Check sheet for the modelled part. Datum: model origin and axes. Units: mm. A direction names the side the tool comes from. Round coordinates to 2 decimals unless told otherwise and drop trailing zeros. Write each loop counter-clockwise with the first axis right and the second up, starting at its lowest first coordinate (ties: lowest second). Pieces come first, ordered by that corner, then holes. Notation, with made-up numbers: M 49.25,-17.5 L 74.25,-17.5 A27 ccw 74.25,2.5 Z; hole C 0.5,9.5 d4. An arc over 180 degrees is marked long. One line per item, written item: value.
from build123d import *

# Parameters (mm, degrees)
SKETCH_R        = 2.5
SKETCH_R_2      = 1.6
PAD_DEPTH       = 65
PAD001_DEPTH    = 1.5
PAD002_DEPTH    = 5
SKETCH003_W     = 2
SKETCH003_H     = 7
POCKET_DEPTH    = 7.001
SKETCH004_R     = 1.1
POCKET001_DEPTH = 7.001
SKETCH006_W     = 2.5
SKETCH006_H     = 11
POCKET002_DEPTH = 8.001
SKETCH005_W     = 2.5
SKETCH005_H     = 11
POCKET003_DEPTH = 8.001
POCKET004_DEPTH = 7.001


with BuildPart() as part:
    # Sketch → Pad (new body)
    with BuildSketch(Plane.XY):
        Circle(SKETCH_R)
        Circle(SKETCH_R_2, mode=Mode.SUBTRACT)
    extrude(amount=PAD_DEPTH)

    # Sketch001 (on Face3 of Pad) → Pad001 (join)
    with BuildSketch(Plane(origin=(0, 0, 7), x_dir=(1, 0, 0), z_dir=(0, 0, -1))):
        with BuildLine():
            Line((-2, 4), (2, 4))
            ThreePointArc((4, 2), (3.414214, 3.414214), (2, 4))
            Line((4, 2), (4, -2))
            ThreePointArc((2, -4), (3.414214, -3.414214), (4, -2))
            Line((2, -4), (-2, -4))
            ThreePointArc((-4, -2), (-3.414214, -3.414214), (-2, -4))
            Line((-4, -2), (-4, 2))
            ThreePointArc((-2, 4), (-3.414214, 3.414214), (-4, 2))
        make_face()
    extrude(amount=-PAD001_DEPTH)

    # Sketch002 (on Face16 of Pad001) → Pad002 (join)
    with BuildSketch(Plane.XY.offset(65)):
        with BuildLine():
            Line((-1, 3), (1, 3))
            ThreePointArc((3, 1), (2.414214, 2.414214), (1, 3))
            Line((3, 1), (3, -1))
            ThreePointArc((1, -3), (2.414214, -2.414214), (3, -1))
            Line((1, -3), (-1, -3))
            ThreePointArc((-3, -1), (-2.414214, -2.414214), (-1, -3))
            Line((-3, -1), (-3, 1))
            ThreePointArc((-1, 3), (-2.414214, 2.414214), (-3, 1))
        make_face()
    extrude(amount=PAD002_DEPTH)

    # Sketch003 (on Face10 of Pad002) → Pocket (cut, through all)
    with BuildSketch(Plane.YZ.offset(3)):
        with Locations((0, 66.5)):
            Rectangle(SKETCH003_W, SKETCH003_H)
    extrude(amount=-POCKET_DEPTH, mode=Mode.SUBTRACT)

    # Sketch004 (on Face3 of Pocket) → Pocket001 (cut, through all)
    with BuildSketch(Plane.XZ.offset(3)):
        with Locations((0, 67.5)):
            Circle(SKETCH004_R)
    extrude(amount=-POCKET001_DEPTH, mode=Mode.SUBTRACT)

    # Sketch006 (on Face28 of Pocket001) → Pocket002 (cut, through all)
    with BuildSketch(Plane.XZ.offset(4)):
        with Locations((0, 16)):
            Rectangle(SKETCH006_W, SKETCH006_H)
        with Locations((0, 29)):
            Rectangle(SKETCH006_W, SKETCH006_H)
        with Locations((0, 42)):
            Rectangle(SKETCH006_W, SKETCH006_H)
        with Locations((0, 55)):
            Rectangle(SKETCH006_W, SKETCH006_H)
    extrude(amount=-POCKET002_DEPTH, mode=Mode.SUBTRACT)

    # Sketch005 (on Face31 of Pocket001) → Pocket003 (cut, through all)
    with BuildSketch(Plane.YZ.offset(4)):
        with Locations((0, 16)):
            Rectangle(SKETCH005_W, SKETCH005_H)
        with Locations((0, 29)):
            Rectangle(SKETCH005_W, SKETCH005_H)
        with Locations((0, 42)):
            Rectangle(SKETCH005_W, SKETCH005_H)
        with Locations((0, 55)):
            Rectangle(SKETCH005_W, SKETCH005_H)
    extrude(amount=-POCKET003_DEPTH, mode=Mode.SUBTRACT)

    # Sketch007 (on Face5 of Pocket003) → Pocket004 (cut, through all)
    with BuildSketch(Plane.XZ.offset(3)):
        with BuildLine():
            ThreePointArc((3, 67.251006), (2.034513, 69.208821), (0, 70))
            Line((0, 70), (3, 70))
            Line((3, 67.251006), (3, 70))
        make_face()
    extrude(amount=-POCKET004_DEPTH, mode=Mode.SUBTRACT)


solid = part.part
Q1. Scan lines: line 1 (Z direction, x = 1, y = 2.5); line 2 (X direction, y = 0, z = 4.75). Record each from-to range of solid material in increasing order. Write a range as [from, to].
Completed:
line 1: [7, 8.5], [65, 67.04], [67.96, 69.83]
line 2: [-2.5, -1.6], [1.6, 2.5]
Q2. Depth check by flat-ended pin: P1, Ø2, axis at x = 0, z = 66.5, coming from the -Y side; P2, Ø0.7, axis at y = -1.5, z = 52.5, coming from the +X side; P3, Ø3, axis at x = -2.5, z = 36.5, coming from the -Y side. Enter the tip coordinate at first touch or a pass-through.
Completed:
P1: y = -3
P2: x = 2.17
P3: y = -2.29
Q3. Sectioned sample at A-A on z = 20.5. Enter the section's corners in (x, y).
Completed:
outline: M -2.17,-1.25 A2.5 ccw -1.25,-2.17 L -1.25,-1.25 Z; M -2.17,1.25 L -1.25,1.25 L -1.25,2.17 A2.5 ccw Z; M 1.25,-2.17 A2.5 ccw 2.17,-1.25 L 1.25,-1.25 Z; M 1.25,1.25 L 2.17,1.25 A2.5 ccw 1.25,2.17 Z
Q4. Sectioned sample at B-B on y = 0. State how many separate pieces and enclosed holes the cut face has, and give its area (3 significant figures).
Completed:
separate pieces: 9
enclosed holes: 0
area: 43.5 mm^2
Q5. Draft check along X on faces 5 (the cylindrical face through (1.669, 1.764, 69.495)), 6 (the cylindrical face through (-2.43, -2.4, 67.46)), 7 (the flat face through (0, 2, 21.5)). Enter one of: pulls with the +X half, pulls with the -X half, needs draft (parallel to the pull), parting line crosses it, or undercut.
Completed:
face 5: pulls with the +X half
face 6: pulls with the -X half
face 7: undercut
Q6. Access from +Z, -Z, +X, -X, +Y, -Y to the whole of each face (thin tool, end or side, straight path). Record for faces 1 (the cylindrical face through (-1.27, -0.97, 3.45)), 2 (the cylindrical face through (-2.4, 2.43, 67.46)), 3 (the flat face through (0, 3, 66)), 4 (the cylindrical face through (-0.208, 1.586, 62.218)).
Completed:
face 1: -Z
face 2: +Z, -X, +Y
face 3: +Z, +X, -X, +Y
face 4: none
